```python
from build123d import *

# Parameters (mm, degrees)
CROQUIS1_R              = 1.5
CROQUIS1_R_2            = 1.55
CROQUIS1_W              = 6.2
CROQUIS1_H              = 30
CROQUIS1_R_3            = 2
CROQUIS1_R_4            = 6.75
CROQUIS1_R_5            = 5.25
SALIENTE_EXTRUIR1_DEPTH = 6


with BuildPart() as part:
    # Croquis1 → Saliente-Extruir1 (new body)
    with BuildSketch(Plane.XY):
        with BuildLine():
            Line((87.635637669, 16), (32.115377174, 16))
            ThreePointArc((32.115377174, 16), (30.701163612, 15.414213562), (30.115377174, 14))
            Line((30.115377174, 14), (30.115377174, 10.910010016))
            Line((30.115377174, 10.910010016), (-30.115377174, 10.910010016))
            Line((-30.115377174, 10.910010016), (-30.115377174, 14))
            ThreePointArc((-30.115377174, 14), (-30.701163612, 15.414213562), (-32.115377174, 16))
            Line((-32.115377174, 16), (-44.664398505, 16))
            Line((-44.664398505, 16), (-87.635637669, 16))
            Line((-87.635637669, 16), (-109, 16))
            ThreePointArc((-109, 16), (-110.414213562, 15.414213562), (-111, 14))
            Line((-111, 14), (-111, 0))
            Line((-111, 0), (-111, -16))
            Line((-111, -16), (-111, -16.087517131))
            ThreePointArc((-111, -16.087517131), (-114.684754838, -37.311709927), (-127.277573278, -54.789258433))
            Line((-127.277573278, -54.789258433), (-135.277573278, -54.789258433))
            Line((-135.277573278, -54.789258433), (-140.277573278, -54.789258433))
            ThreePointArc((-140.277573278, -54.789258433), (-148.762854653, -58.303977059), (-152.277573278, -66.789258433))
            Line((-152.277573278, -66.789258433), (-152.277573278, -304))
            ThreePointArc((-152.277573278, -304), (-148.762854653, -312.485281374), (-140.277573278, -316))
            Line((-140.277573278, -316), (-135.277573278, -316))
            Line((-135.277573278, -316), (-119.364295205, -316))
            Line((-119.364295205, -316), (-96, -316))
            Line((-96, -316), (-44.664398505, -316))
            Line((-44.664398505, -316), (119.364429455, -316))
            Line((119.364429455, -316), (130.295105026, -316))
            Line((130.295105026, -316), (146.942872896, -316))
            ThreePointArc((146.942872896, -316), (155.42815427, -312.485281374), (158.942872896, -304))
            Line((158.942872896, -304), (158.942872896, -70.858545673))
            Line((158.942872896, -70.858545673), (158.942872896, -66.789258433))
            ThreePointArc((158.942872896, -66.789258433), (155.42815427, -58.303977059), (146.942872896, -54.789258433))
            Line((146.942872896, -54.789258433), (126.134028278, -54.789258433))
            ThreePointArc((126.134028278, -54.789258433), (114.918041875, -36.865291264), (111, -16.087517131))
            Line((111, -16.087517131), (111, 14))
            ThreePointArc((111, 14), (110.414213562, 15.414213562), (109, 16))
            Line((109, 16), (87.635637669, 16))
        make_face()
        with Locations((-138.277573278, -306)):
            Circle(CROQUIS1_R, mode=Mode.SUBTRACT)
        with Locations((-95.239711316, -294.840181849)):
            Circle(CROQUIS1_R_2, mode=Mode.SUBTRACT)
        with Locations((-95, -259.840181849)):
            Rectangle(CROQUIS1_W, CROQUIS1_H, mode=Mode.SUBTRACT)
        with Locations((-0.239711316, -294.840181849)):
            Circle(CROQUIS1_R_2, mode=Mode.SUBTRACT)
        with Locations((0, -259.840181849)):
            Rectangle(CROQUIS1_W, CROQUIS1_H, mode=Mode.SUBTRACT)
        with Locations((-95.239711316, -219.840181849)):
            Circle(CROQUIS1_R_2, mode=Mode.SUBTRACT)
        with Locations((-95, -184.840181849)):
            Rectangle(CROQUIS1_W, CROQUIS1_H, mode=Mode.SUBTRACT)
        with Locations((-0.239711316, -219.840181849)):
            Circle(CROQUIS1_R_2, mode=Mode.SUBTRACT)
        with Locations((0, -184.840181849)):
            Rectangle(CROQUIS1_W, CROQUIS1_H, mode=Mode.SUBTRACT)
        with Locations((94.760288684, -294.840181849)):
            Circle(CROQUIS1_R_2, mode=Mode.SUBTRACT)
        with Locations((146.722426722, -306)):
            Circle(CROQUIS1_R, mode=Mode.SUBTRACT)
        with Locations((95, -259.840181849)):
            Rectangle(CROQUIS1_W, CROQUIS1_H, mode=Mode.SUBTRACT)
        with Locations((94.760288684, -219.840181849)):
            Circle(CROQUIS1_R_2, mode=Mode.SUBTRACT)
        with Locations((95, -184.840181849)):
            Rectangle(CROQUIS1_W, CROQUIS1_H, mode=Mode.SUBTRACT)
        with Locations((-95.239711316, -144.840181849)):
            Circle(CROQUIS1_R_2, mode=Mode.SUBTRACT)
        with Locations((-95, -109.840181849)):
            Rectangle(CROQUIS1_W, CROQUIS1_H, mode=Mode.SUBTRACT)
        with Locations((-95.239711316, -69.840181849)):
            Circle(CROQUIS1_R_2, mode=Mode.SUBTRACT)
        with Locations((-0.239711316, -144.840181849)):
            Circle(CROQUIS1_R_2, mode=Mode.SUBTRACT)
        with Locations((0, -109.840181849)):
            Rectangle(CROQUIS1_W, CROQUIS1_H, mode=Mode.SUBTRACT)
        with Locations((-0.239711316, -69.840181849)):
            Circle(CROQUIS1_R_2, mode=Mode.SUBTRACT)
        with Locations((-138.277573278, -61)):
            Circle(CROQUIS1_R, mode=Mode.SUBTRACT)
        with Locations((-95, -34.840181849)):
            Rectangle(CROQUIS1_W, CROQUIS1_H, mode=Mode.SUBTRACT)
        with Locations((-106.313708499, -11.313708499)):
            Circle(CROQUIS1_R_3, mode=Mode.SUBTRACT)
        with Locations((-83.686291501, -11.313708499)):
            Circle(CROQUIS1_R_3, mode=Mode.SUBTRACT)
        with Locations((-95, 0)):
            Circle(CROQUIS1_R_4, mode=Mode.SUBTRACT)
        with Locations((-106.313708499, 11.313708499)):
            Circle(CROQUIS1_R_3, mode=Mode.SUBTRACT)
        with Locations((-83.686291501, 11.313708499)):
            Circle(CROQUIS1_R_3, mode=Mode.SUBTRACT)
        with Locations((0, -34.840181849)):
            Rectangle(CROQUIS1_W, CROQUIS1_H, mode=Mode.SUBTRACT)
        with Locations((-5.656854249, -5.656854249)):
            Circle(CROQUIS1_R, mode=Mode.SUBTRACT)
        Circle(CROQUIS1_R_5, mode=Mode.SUBTRACT)
        with Locations((-5.656854249, 5.656854249)):
            Circle(CROQUIS1_R, mode=Mode.SUBTRACT)
        with Locations((94.760288684, -144.840181849)):
            Circle(CROQUIS1_R_2, mode=Mode.SUBTRACT)
        with Locations((95, -109.840181849)):
            Rectangle(CROQUIS1_W, CROQUIS1_H, mode=Mode.SUBTRACT)
        with Locations((94.760288684, -69.840181849)):
            Circle(CROQUIS1_R_2, mode=Mode.SUBTRACT)
        with Locations((5.656854249, -5.656854249)):
            Circle(CROQUIS1_R, mode=Mode.SUBTRACT)
        with Locations((5.656854249, 5.656854249)):
            Circle(CROQUIS1_R, mode=Mode.SUBTRACT)
        with Locations((95, -34.840181849)):
            Rectangle(CROQUIS1_W, CROQUIS1_H, mode=Mode.SUBTRACT)
        with Locations((146.722426722, -61)):
            Circle(CROQUIS1_R, mode=Mode.SUBTRACT)
        with Locations((83.686291501, -11.313708499)):
            Circle(CROQUIS1_R_3, mode=Mode.SUBTRACT)
        with Locations((106.313708499, -11.313708499)):
            Circle(CROQUIS1_R_3, mode=Mode.SUBTRACT)
        with Locations((95, 0)):
            Circle(CROQUIS1_R_4, mode=Mode.SUBTRACT)
        with Locations((83.686291501, 11.313708499)):
            Circle(CROQUIS1_R_3, mode=Mode.SUBTRACT)
        with Locations((106.313708499, 11.313708499)):
            Circle(CROQUIS1_R_3, mode=Mode.SUBTRACT)
    extrude(amount=SALIENTE_EXTRUIR1_DEPTH)


solid = part.part
```
Could you check a few things on this model? Use its own coordinates, in mm. Give positions to 0.01 mm unless a question says otherwise; leave off trailing zeros. Loops run counter-clockwise (first coordinate to the right, second up) from the corner with the lowest first, then second, coordinate; pieces in that order, holes last. Notation, with made-up numbers: (-36, -0.75) - (-5, -0.75) arc R9 cw to (-5, 14.25) - close; hole circle Ø2 at (-39, -12). An arc over 180 degrees is marked (long way). Answer in a Markdown table with one row per item. Add a question column.
Q1. Please list where these lines run through material, in increasing order: L1, parallel to X at y = -115.5, z = 2.2; L2, parallel to X at y = -5.5, z = 1.15; L3, parallel to X at y = -27, z = 2.1. Write a range as from..to.
Q2. We'd pull the mould along Y, two halves only. Please class faces 1 (the face through (-88.765, -2.585, 2.958)), 2 (the face through (115.027, -37.142, 2.958)), 3 (the face through (-148.856, -312.391, 2.958)): +Y half, -Y half, draft (parallel to the pull), parting line (faces both ways), or undercut.
Q3. If we section it at A-A (y = 0): List the corners of the cut face in (x, z) for me, plus the area to 3 significant figures.
Q4. For pin 1 (0.9 mm diameter, centred on y = 12.5, z = 3.5, fed in from -X); pin 2 (3 mm diameter, centred on x = -83.69, y = -11.31, fed in from +Z); pin 3 (3 mm diameter, centred on x = 133, z = 4, fed in from +Y), each with a flat end and sliding along its axis, tell me the tip position at first contact or that it passes through.
Q5. If we section it at B-B (x = -132): List the corners of the cut face in (y, z) for me, plus the area to 3 significant figures.
Q6. If we section it at C-C (z = 3.05): State how many separate pieces and enclosed holes the cut face has, plus the area to 3 significant figures.
The answers:
| question | item | result |
|---|---|---|
| 1 | L1 | x = -152.28..-98.1, -91.9..-3.1, 3.1..91.9, 98.1..158.94 |
| 1 | L2 | x = -111..-98.91, -91.09..-7.15, -4.17..4.17, 7.15..91.09, 98.91..111 |
| 1 | L3 | x = -111.65..-98.1, -91.9..-3.1, 3.1..91.9, 98.1..112.05 |
| 2 | face 1 | undercut |
| 2 | face 2 | +Y half |
| 2 | face 3 | -Y half |
| 3 | outline | (-111, 0) - (-101.75, 0) - (-101.75, 6) - (-111, 6) - close; (-88.25, 0) - (-5.25, 0) - (-5.25, 6) - (-88.25, 6) - close; (5.25, 0) - (88.25, 0) - (88.25, 6) - (5.25, 6) - close; (101.75, 0) - (111, 0) - (111, 6) - (101.75, 6) - close |
| 3 | area | 1,110 mm^2 |
| 4 | pin 1 | stops at x = -111 |
| 4 | pin 2 | passes through |
| 4 | pin 3 | stops at y = -54.79 |
| 5 | outline | (-316, 0) - (-54.79, 0) - (-54.79, 6) - (-316, 6) - close |
| 5 | area | 1,570 mm^2 |
| 6 | separate pieces | 1 |
| 6 | enclosed holes | 43 |
| 6 | area | 94,100 mm^2 |
